```python
from build123d import *

# Parameters (mm, degrees)
F0_W     = 5.352506
F0_H     = 1.93545
F1_DEPTH = 25.4
F2_R     = 2.286
F3_R     = 1.907129
F4_DEPTH = 2.39776


with BuildPart() as f1:
    # F0 (on Front) → F1 (new body)
    with BuildSketch(Plane.XZ):
        Rectangle(F0_W, F0_H)
    extrude(amount=F1_DEPTH)

    # F2
    f2_edges = [f1.edges().sort_by_distance(p)[0] for p in [
        (-2.676253, -25.4, 0),
        (2.676253, -25.4, 0),
    ]]
    fillet(f2_edges, radius=F2_R)

    # F3 (on face) → F4 (cut)
    with BuildSketch(Plane.XY.offset(0.967725)):
        with Locations((0, -21.805298)):
            Circle(F3_R)
    extrude(amount=-F4_DEPTH, mode=Mode.SUBTRACT)


solid = f1.part
```
Could you check a few things on this model? Use its own coordinates, in mm. Coordinates: 2 decimals unless noted, no trailing zeros. Loops run counter-clockwise (first coordinate to the right, second up) from the corner with the lowest first, then second, coordinate; pieces in that order, holes last. Notation, with made-up numbers: M 27.25,37.25 L 69.25,37.25 A24 ccw 69.25,76.25 Z; hole C 21.5,60 d1. An arc over 180 degrees is marked long. Put each result on its own line as item: value. Start each with the question number.
(1) I need wall thicknesses on line 1 (Y direction, x = 0, z = -0.5); line 2 (Y direction, x = 1.45, z = 0.45); line 3 (Y direction, x = -2.1, z = 0.4). Which ranges of each line are inside material? Lowest first, please. Write a range as from..to.
(2) Suppose I cut it at C-C on y = -20.5. Please give me the cut outline in (x, z).
(3) Suppose I cut it at A-A on x = 0. Please give me the cut outline in (y, z), then the cut area to 3 significant figures.
(4) Suppose I cut it at B-B on z = 0.3. Please give me the cut outline in (x, y), then the cut area to 3 significant figures.
Solutions:
1. line 1: y = -25.4..-23.71, -19.9..0
1. line 2: y = -25.14..-23.04, -20.57..0
1. line 3: y = -24.63..0
2. outline: M -2.68,-0.97 L -1.39,-0.97 L -1.39,0.97 L -2.68,0.97 Z; M 1.39,-0.97 L 2.68,-0.97 L 2.68,0.97 L 1.39,0.97 Z
3. outline: M -25.4,-0.97 L -23.71,-0.97 L -23.71,0.97 L -25.4,0.97 Z; M -19.9,-0.97 L 0,-0.97 L 0,0.97 L -19.9,0.97 Z
3. area: 41.8 mm2
4. outline: M -2.68,-23.11 A2.29 ccw -0.39,-25.4 L 0.39,-25.4 A2.29 ccw 2.68,-23.11 L 2.68,0 L -2.68,0 Z; hole C 0,-21.81 d3.81
4. area: 122 mm2
